```python
from build123d import *

# Parameters (mm, degrees)
BOSS_EXTRUDE1_DEPTH = 1.016
SKETCH2_R           = 0.635
SKETCH2_R_2         = 0.381
CUT_EXTRUDE1_DEPTH  = 20.63947316


with BuildPart() as part:
    # Sketch1 → Boss-Extrude1 (new body)
    with BuildSketch(Plane(origin=(0, 0, 0), x_dir=(1, 0, 0), z_dir=(0, 1, 0))):
        with BuildLine():
            Line((0, 0), (8.255, 0))
            Line((8.255, 0), (8.255, 4.9276))
            Line((8.255, 4.9276), (9.525, 4.9276))
            Line((9.525, 4.9276), (-2.539137852, 16.669908865))
            ThreePointArc((-2.539137852, 16.669908865), (-4.360383855, 17.013020284), (-5.3848, 15.4686))
            Line((-5.3848, 15.4686), (-5.3848, 11.8618))
            Line((-5.3848, 11.8618), (-1.524, 4.9276))
            Line((-1.524, 4.9276), (0, 4.9276))
            Line((0, 4.9276), (0, 0))
        make_face()
    extrude(amount=BOSS_EXTRUDE1_DEPTH)

    # Sketch2 → Cut-Extrude1 (cut, through all)
    with BuildSketch(Plane(origin=(0, 1.016, 0), x_dir=(1, 0, 0), z_dir=(0, 1, 0))):
        with Locations(Location((-3.4798, 15.0368, 0), (0, 0, 270))):
            Circle(SKETCH2_R)
        with Locations(Location((-3.4798, 13.0302, 0), (0, 0, 270))):
            Circle(SKETCH2_R_2)
    extrude(amount=-CUT_EXTRUDE1_DEPTH, mode=Mode.SUBTRACT)


solid = part.part
```
Model file for the job. Use its own axes, mm. A direction names the side the tool comes from. Coordinates: 2 decimals unless noted, no trailing zeros. Loops run counter-clockwise (first coordinate to the right, second up) from the corner with the lowest first, then second, coordinate; pieces in that order, holes last. Notation, with made-up numbers: M 11,68 L 50,68 A4 cw 50,73 Z; hole C 30,33.5 d8. An arc over 180 degrees is marked long. Use CSV: the item, a comma, the result in double quotes. Start each with the question number.
1. Tool access for faces 1 (the flat face through (8.9, 0.5, -4.928)), 2 (the flat face through (0, 0.5, -2.5)), 3 (the flat face through (4.1, 0.5, 0)): list every direction of +Z, -Z, +X, -X, +Y, -Y with a clear straight run to the whole face (end or side of a thin tool).
2. Probe probe 1 along X at (y, z) = (0.5, -14.75); probe 2 along X at (y, z) = (0.45, -3.25) (3 decimals); probe 3 along Z at (x, y) = (-4, 0.9). List the from-to ranges inside material, lowest first. Write a range as [from, to].
3. Band-saw the part on A-A, the plane z = -15.25. List the corners of the cut face in (x, y).
4. Band-saw the part on D-D, the plane x = 4.5. List the corners of the cut face in (y, z), then the cut area to 3 significant figures.
5. Band-saw the part on B-B, the plane y = 0.6. List the corners of the cut face in (x, z) (3 decimals).
6. Two-plate mould, pull along Z, no slides. Class faces 4 (the cylindrical face through (-3.45, 0.52, -15.67)), 5 (the flat face through (-5.385, 0.5, -13.7)), 6 (the flat face through (3.577, 0.501, -10.717)): pulls with the +Z half, pulls with the -Z half, needs draft (parallel to the pull), parting line crosses it, or undercut.
7. Band-saw the part on C-C, the plane x = 0.5. List the corners of the cut face in (y, z).
Entries:
1,face 1,"+Z, +X, +Y, -Y"
1,face 2,"+Z, -X, +Y, -Y"
1,face 3,"+Z, +X, -X, +Y, -Y"
2,probe 1,"x = [-5.38, -4.05], [-2.91, -0.57]"
2,probe 2,"x = [0, 8.255]"
2,probe 3,"z = [-17.12, -15.4], [-14.67, -9.37]"
3,outline,"M -5.38,0 L -4.08,0 L -4.08,1.02 L -5.38,1.02 Z; M -2.88,0 L -1.08,0 L -1.08,1.02 L -2.88,1.02 Z"
4,outline,"M 0,-9.82 L 1.02,-9.82 L 1.02,0 L 0,0 Z"
4,area,"9.98 mm2"
5,outline,"M -5.385,-15.469 A1.676 ccw -2.539,-16.67 L 9.525,-4.928 L 8.255,-4.928 L 8.255,0 L 0,0 L 0,-4.928 L -1.524,-4.928 L -5.385,-11.862 Z; hole C -3.48,-15.037 d1.27; hole C -3.48,-13.03 d0.762"
6,face 4,"undercut"
6,face 5,"needs draft"
6,face 6,"pulls with the -Z half"
7,outline,"M 0,-13.71 L 1.02,-13.71 L 1.02,0 L 0,0 Z"
